Geometry: final body of the model. Coordinates: model frame, mm. A direction names the side the tool comes from. Give positions to 0.01 mm unless a question says otherwise; leave off trailing zeros. Order: outer loops, then holes, each group sorted by start corner. A loop starts at its lowest first (then second) coordinate and runs counter-clockwise, first axis right, second up. Notation, with made-up numbers: (54, 11) - (83, 11) arc R18 cw to (83, 29) - close; hole circle Ø11 at (49.25, 66). An arc over 180 degrees is marked (long way). One line per item, written item: value.
Autodesk Inventor part; units mm, degrees
ref_plane "YZ Plane" through (0, 0, 0) normal (1, 0, 0) x (0, 1, 0)
ref_plane "XZ Plane" through (0, 0, 0) normal (0, 1, 0) x (-1, 0, 0)
ref_plane "XY Plane" through (0, 0, 0) normal (0, 0, 1) x (1, 0, 0)
sketch "Sketch1" plane through (0, 0, 0) normal (0, 0, 1) x (1, 0, 0)
  circle A0 centre (0, 0) radius 35
  dimension "d0" = 70
extrude "Extrusion1" add sketch "Sketch1" along normal mid plane 50
sketch "Sketch2" plane through (0, 0, 0) normal (0, 0, 1) x (1, 0, 0)
  circle A0 centre (0, 0) radius 35
  line L0 (0, -35) -> (25, -35)
  line L1 (25, -35) -> (25, -24.4949)
  arc A1 (0, -35) -> (25, -24.4949) centre (0, 0) ccw
  line L2 (25, -24.4949) -> (-25, -24.4949)
  line L3 (-25, -35) -> (0, -35)
  line L4 (-25, -35) -> (-25, -24.4949)
  arc A2 (-25, -24.4949) -> (0, -35) centre (0, 0) ccw
  dimension "d3" = 25
  dimension "d6" = 25
extrude "Extrusion2" add sketch "Sketch2" along normal mid plane 50
sketch "Sketch4" plane through (-25, -35, 25) normal (0, -1, 0) x (1, 0, 0)
  circle A0 centre (25, -25) radius 12.5
  dimension "d7" = 25
extrude "Extrusion3" cut sketch "Sketch4" against normal blind 10
1) Section A-A, the plane z = 10.5. Return loops of the section in (x, y).
Answers below:
outline: (-25, -35) - (-6.78, -35) - (-6.78, -25) - (6.78, -25) - (6.78, -35) - (25, -35) - (25, -24.49) arc R35 ccw (long way) to (-25, -24.49) - close
2) Section C-C, the plane y = -10. Return loops of the section in (x, z), then the cut area to 3 significant figures.
Answers below:
outline: (-33.54, -25) - (33.54, -25) - (33.54, 25) - (-33.54, 25) - close
area: 3,350 mm^2
3) Section D-D, the plane z = -17.5. Return loops of the section in (x, y).
Answers below:
outline: (-25, -35) - (25, -35) - (25, -24.49) arc R35 ccw (long way) to (-25, -24.49) - close
4) Material intervals for line 1 along Z through (x, y) = (3, -25.5); line 2 along X through (y, z) = (0.5, -4); line 3 along X through (y, z) = (-6, -18), sorted ascending.
Answers below:
line 1: -25 to -12.13, 12.13 to 25
line 2: -35 to 35
line 3: -34.48 to 34.48
5) Set-up query: faces 1 (the face through (11.923, -30.07, 3.755)), 2 (the face through (-5.9, -35, -11.5)), 3 (the face through (25, -30, 0)), 4 (the face through (-25, -30, 0)). Return all of +Z, -Z, +X, -X, +Y, -Y with unobstructed straight access to the full face (end or side cutting, diameter ignored); none if empty.
Answers below:
face 1: -Y
face 2: +Z, -Z, +X, -X, -Y
face 3: +Z, -Z, +X, -Y
face 4: +Z, -Z, -X, -Y
6) Section B-B, the plane x = 0. Return loops of the section in (y, z), then the cut area to 3 significant figures.
Answers below:
outline: (-35, -25) - (35, -25) - (35, 25) - (-35, 25) - (-35, 12.5) - (-25, 12.5) - (-25, -12.5) - (-35, -12.5) - close
area: 3,250 mm^2
7) First-contact query: pin 1 (1.5 mm diameter, centred on y = 13.5, z = 15.5, fed in from -X); pin 2 (2 mm diameter, centred on x = 0, z = -1.5, fed in from -Y); pin 3 (2 mm diameter, centred on y = -7, z = -13, fed in from -X). Flat tips, straight axial feed; report the tip coordinate or a pass-through.
Answers below:
pin 1: x = -32.6
pin 2: y = -25
pin 3: x = -34.48
